Geometry: final body of the model. Coordinates: model frame, mm. A direction names the side the tool comes from. Round coordinates to 2 decimals unless told otherwise and drop trailing zeros. Order: outer loops, then holes, each group sorted by start corner. A loop starts at its lowest first (then second) coordinate and runs counter-clockwise, first axis right, second up. Notation, with made-up numbers: M 61.25,88.25 L 115.25,88.25 A30 cw 115.25,115.25 Z; hole C 52,51.5 d4. An arc over 180 degrees is marked long. Put each result on its own line as item: value. Start each with the question number.
1) Material intervals for probe 1 along X at (y, z) = (10, 1.2); probe 2 along X at (y, z) = (14, 3.5); probe 3 along X at (y, z) = (18.5, 0.3), sorted ascending. Write a range as [from, to].
2) Access query for faces 1 (the flat face through (91, 10, 6)), 2 (the flat face through (11.5, 10, 3)). Directions: +Z, -Z, +X, -X, +Y, -Y. A direction counts if a zero-diameter tool reaches every point of the face in a straight line with its end or side. Return the directions, or none.
3) Draft query along Y for faces 3 (the flat face through (8.5, 10, 3)), 4 (the cylindrical face through (2.85, 16.99, 3.04)), 5 (the flat face through (91, 10, 0)), 6 (the flat face through (10, 8.5, 3)). Return one class per face: pulls with the +Y half, pulls with the -Y half, needs draft (parallel to the pull), parting line crosses it, or undercut.
4) Section A-A, the plane y = 17. Return loops of the section in (x, z).
from build123d import *

# Parameters (mm, degrees)
SKETCH1_W           = 185
SKETCH1_H           = 20
BOSS_EXTRUDE1_DEPTH = 6
SKETCH2_W           = 3
SKETCH2_H           = 3
CUT_EXTRUDE2_DEPTH  = 187.174649187
FILLET1_R           = 10


with BuildPart() as part:
    # Sketch1 → Boss-Extrude1 (new body)
    with BuildSketch(Plane.XY):
        with Locations((92.5, 10)):
            Rectangle(SKETCH1_W, SKETCH1_H)
    extrude(amount=BOSS_EXTRUDE1_DEPTH)

    # Sketch2 → Cut-Extrude2 (cut, through all)
    with BuildSketch(Plane.XY.offset(6)):
        with Locations((10, 10)):
            Rectangle(SKETCH2_W, SKETCH2_H)
    extrude(amount=-CUT_EXTRUDE2_DEPTH, mode=Mode.SUBTRACT)

    # Fillet1
    fillet1_edges = [part.edges().sort_by_distance(p)[0] for p in [
        (0, 0, 3),
        (0, 20, 3),
    ]]
    fillet(fillet1_edges, radius=FILLET1_R - 0.0001)  # a hair under: the kernel refuses the full size


solid = part.part
Result sheet:
1. probe 1: x = [0, 8.5], [11.5, 185]
1. probe 2: x = [0.83, 185]
1. probe 3: x = [4.73, 185]
2. face 1: +Z, +X, -X, +Y, -Y
2. face 2: +Z, -Z
3. face 3: undercut
3. face 4: pulls with the +Y half
3. face 5: needs draft
3. face 6: undercut
4. outline: M 2.86,0 L 185,0 L 185,6 L 2.86,6 Z
